Here's how the part is built. I have some questions about the finished solid (model axes, mm). A direction names the side the tool comes from. Give positions to 0.01 mm unless a question says otherwise; leave off trailing zeros. Order: outer loops, then holes, each group sorted by start corner. A loop starts at its lowest first (then second) coordinate and runs counter-clockwise, first axis right, second up. Notation, with made-up numbers: M -7,-8 L 42,-8 A17 ccw 42,-4 Z; hole C 55,49.25 d7. An arc over 180 degrees is marked long. Use one line per item in the form item = value.
from build123d import *

# Parameters (mm, degrees)
SKETCH1_R           = 3.5
BOSS_EXTRUDE1_DEPTH = 10
SKETCH2_R           = 3
CUT_EXTRUDE1_DEPTH  = 9
SKETCH3_R           = 0.5
BOSS_EXTRUDE2_DEPTH = 9
FILLET1_R           = 0.5
SKETCH4_W           = 10
SKETCH4_H           = 10
BOSS_EXTRUDE3_DEPTH = 1


with BuildPart() as part:
    # Sketch1 → Boss-Extrude1 (new body)
    with BuildSketch(Plane(origin=(0, 0, 0), x_dir=(1, 0, 0), z_dir=(0, 1, 0))):
        with Locations(Location((0, 0, 0), (0, 0, 270))):
            Circle(SKETCH1_R)
    extrude(amount=BOSS_EXTRUDE1_DEPTH)

    # Sketch2 → Cut-Extrude1 (cut)
    with BuildSketch(Plane(origin=(0, 10, 0), x_dir=(1, 0, 0), z_dir=(0, 1, 0))):
        with Locations(Location((0, 0, 0), (0, 0, 270))):
            Circle(SKETCH2_R)
    extrude(amount=-CUT_EXTRUDE1_DEPTH, mode=Mode.SUBTRACT)

    # Sketch3 → Boss-Extrude2 (add)
    with BuildSketch(Plane(origin=(0, 1, 0), x_dir=(1, 0, 0), z_dir=(0, 1, 0))):
        with Locations(Location((0, 0, 0), (0, 0, 270))):
            Circle(SKETCH3_R)
    extrude(amount=BOSS_EXTRUDE2_DEPTH)

    # Fillet1
    fillet1_edges = [part.edges().sort_by_distance(p)[0] for p in [
        (0, 10, -0.5),
        (0, 10, -3),
    ]]
    fillet(fillet1_edges, radius=FILLET1_R - 0.0001)  # a hair under: the kernel refuses the full size

    # Sketch4 → Boss-Extrude3 (add)
    with BuildSketch(Plane(origin=(0, 0, 0), x_dir=(-1, 0, 0), z_dir=(0, -1, 0))):
        Rectangle(SKETCH4_W, SKETCH4_H)
    extrude(amount=BOSS_EXTRUDE3_DEPTH)


solid = part.part
Q1. On a 3-axis mill with a long thin cutter (end or side, diameter ignored), from which of +Z, -Z, +X, -X, +Y, -Y can I reach the whole of each face in a straight line? I mean faces 1 (the face through (0, -1, 0)), 2 (the face through (0.9, 5.31, 2.86)). Say none if no direction works.
Found:
face_1 = +Z, -Z, +X, -X, -Y
face_2 = +Y
Q2. I need wall thicknesses on L1, parallel to X at y = 7.75, z = 0; L2, parallel to Y at x = 1.25, z = -4.25; L3, parallel to Z at x = -0.25, y = 3. Which ranges of each line are inside material? Lowest first, please.
Found:
L1 = -3.5 to -3, -0.5 to 0.5, 3 to 3.5
L2 = -1 to 0
L3 = -3.49 to -2.99, -0.43 to 0.43, 2.99 to 3.49
Q3. I want a section at A-A on y = 8.25. Write out the boundary of the cut face in (x, z).
Found:
outline = C 0,0 d7; C 0,0 d1; hole C 0,0 d6
Q4. Thinking about a two-plate mould opening in X: for faces 3 (the face through (5, -0.5, 0.1)), 4 (the face through (-5, -0.5, 0.1)), 5 (the face through (-0.488, 5.191, -0.108)), which applies, +X half, -X half, draft (parallel to the pull), parting line (faces both ways), or undercut?
Found:
face_3 = +X half
face_4 = -X half
face_5 = undercut
Q5. I'm going to push flat-ended pins straight in: pin 1 Ø4 at (x, y) = (4, 7.5) entering from -Z; pin 2 Ø3 at (y, z) = (2.5, -2.5) entering from +X; pin 3 Ø5 at (y, z) = (6, 4) entering from -X. Where does each tip first touch, or does it pass through?
Found:
pin_1 = -2.87
pin_2 = 3.35
pin_3 = -3.16
